Here's the drawing with two shaded views (mm, measured from the low corner). I have some questions. Round coordinates to 2 decimals unless told otherwise and drop trailing zeros. Order: outer loops, then holes, each group sorted by start corner. A loop starts at its lowest first (then second) coordinate and runs counter-clockwise, first axis right, second up. Notation, with made-up numbers: (51, -21.5) -> (93, -21.5) arc R20 cw to (93, 0.5) -> close; hole circle Ø9 at (29.25, -23). An arc over 180 degrees is marked (long way). Put each result on its own line as item: value. Start each with the question number.
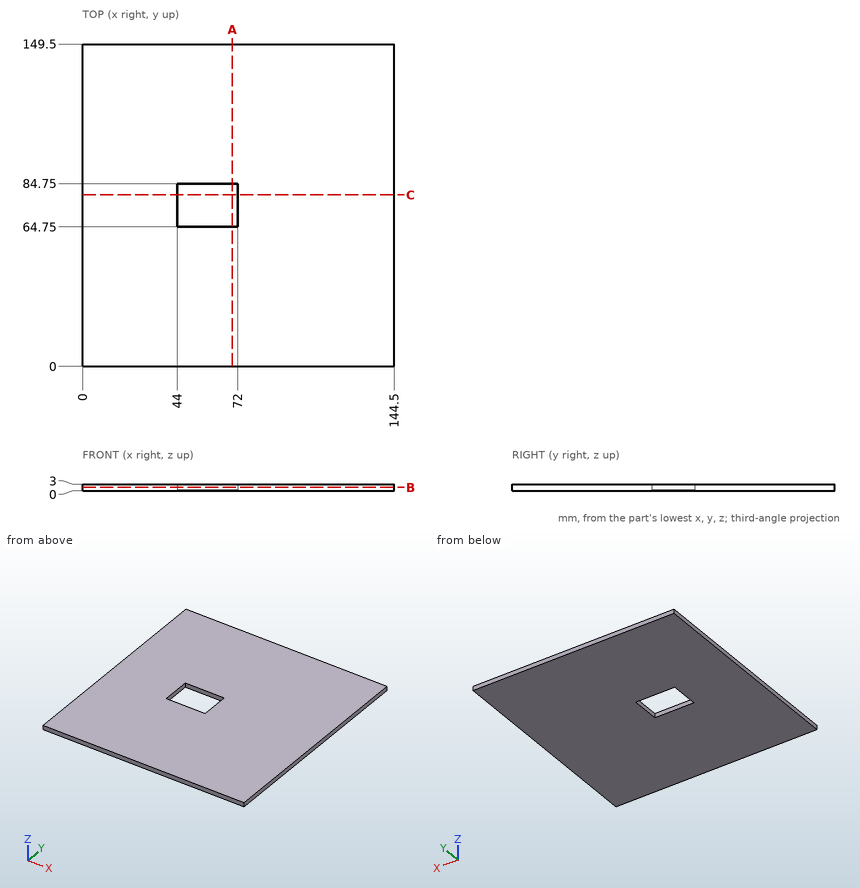
1. If we section it at A-A, the plane x = 69.5: Please give me the cut outline in (y, z), then the cut area to 4 significant figures.
2. If we section it at C-C, the plane y = 79.5: Please give me the cut outline in (x, z).
3. If we section it at B-B, the plane z = 1.65: Please give me the cut outline in (x, y), then the cut area to 3 significant figures.
4. I need wall thicknesses on L1, parallel to Y at x = 48, z = 2.25; L2, parallel to X at y = 75, z = 1.2. Which ranges of each line are inside material? Lowest first, please.
Results below:
1. outline: (0, 0) -> (64.75, 0) -> (64.75, 3) -> (0, 3) -> close; (84.75, 0) -> (149.5, 0) -> (149.5, 3) -> (84.75, 3) -> close
1. area: 388.5 mm2
2. outline: (0, 0) -> (44, 0) -> (44, 3) -> (0, 3) -> close; (72, 0) -> (144.5, 0) -> (144.5, 3) -> (72, 3) -> close
3. outline: (0, 0) -> (144.5, 0) -> (144.5, 149.5) -> (0, 149.5) -> close; hole (44, 64.75) -> (72, 64.75) -> (72, 84.75) -> (44, 84.75) -> close
3. area: 21,000 mm2
4. L1: 0 to 64.75, 84.75 to 149.5
4. L2: 0 to 44, 72 to 144.5
